Could you check a few things on this model? Use its own coordinates, in mm. A direction names the side the tool comes from. Give positions to 0.01 mm unless a question says otherwise; leave off trailing zeros. Loops run counter-clockwise (first coordinate to the right, second up) from the corner with the lowest first, then second, coordinate; pieces in that order, holes last. Notation, with made-up numbers: M 46.5,-34.5 L 76.5,-34.5 A19 cw 76.5,1.5 Z; hole C 39,5.5 d9. An arc over 180 degrees is marked long. Answer in a Markdown table with one row per item. Add a question column.
```python
from build123d import *

# Parameters (mm, degrees)
SKETCH1_W          = 9.525
SKETCH1_H          = 1.4224
CHAMFER1_SIZE      = 0.47625
SKETCH4_R          = 2.7051
EXTRUDE1_DEPTH     = 1.4986
CUT_EXTRUDE1_DEPTH = 0.7493
SKETCH7_R          = 0.916543552
CUT_EXTRUDE4_DEPTH = 0.7493
CUT_EXTRUDE4_TAPER = 45
SKETCH8_R          = 0.79375
CUT_EXTRUDE5_DEPTH = 0.249766667
CUT_EXTRUDE5_TAPER = 60


with BuildPart() as part:
    # Sketch1 → Revolve1 (revolve)
    with BuildSketch(Plane(origin=(0, 0, 0), x_dir=(0, 0, -1), z_dir=(1, 0, 0))):
        with Locations((4.7625, 0.7112)):
            Rectangle(SKETCH1_W, SKETCH1_H)
    revolve(axis=Axis((0, 0, 0), (0, 0, 1)))

    # Chamfer1
    chamfer1_edges = [part.edges().sort_by_distance(p)[0] for p in [
        (0, -1.4224, -9.525),
    ]]
    chamfer(chamfer1_edges, length=CHAMFER1_SIZE)

    # Sketch4 → Extrude1 (add)
    with BuildSketch(Plane.XY):
        Circle(SKETCH4_R)
    extrude(amount=EXTRUDE1_DEPTH)

    # Sketch9 → Cut-Revolve3 (revolve, cut)
    with BuildSketch(Plane(origin=(0, 0, 0), x_dir=(0, 0, -1), z_dir=(1, 0, 0))):
        with BuildLine():
            Line((0, 2.7051), (-0.381, 2.7051))
            ThreePointArc((-0.381, 2.7051), (-1.025093234, 2.138064897), (-1.4986, 1.4224))
            Line((-1.4986, 1.4224), (-1.8796, 1.4224))
            Line((-1.8796, 1.4224), (-1.8796, 3.0861))
            Line((-1.8796, 3.0861), (0, 3.0861))
            Line((0, 3.0861), (0, 2.7051))
        make_face()
    revolve(axis=Axis((0, 0, 0), (0, 0, 1)), mode=Mode.SUBTRACT)

    # Sketch6 → Cut-Extrude1 (cut)
    with BuildSketch(Plane.XY.offset(1.4986)):
        Polygon((0, -0.916543552), (0.79375, -0.458271776), (0.79375, 0.458271776), (0, 0.916543552), (-0.79375, 0.458271776), (-0.79375, -0.458271776), align=None)
    extrude(amount=-CUT_EXTRUDE1_DEPTH, mode=Mode.SUBTRACT)

    # Sketch7 → Cut-Extrude4 (cut)
    with BuildSketch(Plane.XY.offset(1.4986)):
        Circle(SKETCH7_R)
    extrude(amount=-CUT_EXTRUDE4_DEPTH, taper=CUT_EXTRUDE4_TAPER, mode=Mode.SUBTRACT)

    # Sketch8 → Cut-Extrude5 (cut)
    with BuildSketch(Plane.XY.offset(0.7493)):
        Circle(SKETCH8_R)
    extrude(amount=-CUT_EXTRUDE5_DEPTH, taper=CUT_EXTRUDE5_TAPER, mode=Mode.SUBTRACT)


solid = part.part
```
Item 1: I need wall thicknesses on L1, parallel to Z at x = -1.05, y = -0.15; L2, parallel to X at y = 0.85, z = -3.25; L3, parallel to X at y = 1, z = 0.5. Which ranges of each line are inside material? Lowest first, please.
Item 2: Suppose I cut it at A-A (z = -3.25). List the corners of the cut face in (x, y) for me.
Item 3: For faces 1 (the face through (1.2, -1.2, 0)), 2 (the face through (2.499, -1.036, 0.188)), which set-ups out of +Z, -Z, +X, -X, +Y, -Y let a thin tool reach every point of the face, with its end or its side?
Item 4: For P1, Ø1.5, axis at x = -2, y = 1.5, coming from the -Z side; P2, Ø1.5, axis at x = 1.5, y = 0.5, coming from the +Z side; P3, Ø0.6, axis at y = 0, z = 1.5, coming from the +X side; P4, Ø0.8, axis at y = 0, z = 1, coming from the -X side (3 decimals), each with a flat end and sliding along its axis, tell me the tip position at first contact or that it passes through.
Item 5: Suppose I cut it at B-B (y = -1.95). List the corners of the cut face in (x, z) for me.
Item 6: Suppose I cut it at C-C (x = -1.65). List the corners of the cut face in (y, z) for me, then the cut area to 3 significant figures.
Values found:
| question | item | result |
|---|---|---|
| 1 | L1 | -9.41 to 1.5 |
| 1 | L2 | -1.14 to 1.14 |
| 1 | L3 | -2.42 to 2.42 |
| 2 | outline | C 0,0 d2.84 |
| 3 | face 1 | -Z |
| 3 | face 2 | +Z, -Z |
| 4 | P1 | z = 0 |
| 4 | P2 | z = 1.5 |
| 4 | P3 | x = 1.92 |
| 4 | P4 | x = -2.545 |
| 5 | outline | M -1.87,0 L 1.87,0 L 1.87,0.38 A2.61 ccw -1.87,0.38 Z |
| 6 | outline | M -2.14,0 L 2.14,0 L 2.14,0.38 A2.81 ccw -2.14,0.38 Z |
| 6 | area | 4.60 mm² |
